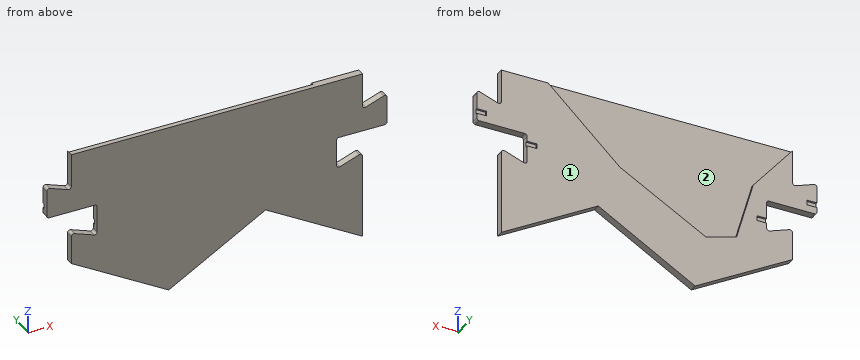
```python
from build123d import *

# Parameters (mm, degrees)
P_IDAT_VYSUNUT_M1_DEPTH  = 3
P_IDAT_VYSUNUT_M2_DEPTH  = 2
ZAOBLIT3_R               = 1
SKICA2_W                 = 4
SKICA2_H                 = 2
ODEBRAT_VYSUNUT_M1_DEPTH = 0.8
SKICA3_W                 = 4
SKICA3_H                 = 2
ODEBRAT_VYSUNUT_M2_DEPTH = 0.8


with BuildPart() as part:
    # Skica1 → P_idat vysunut_m1 (new body)
    with BuildSketch(Plane(origin=(0, 0, 0), x_dir=(1, 0, 0), z_dir=(0, 1, 0))):
        Polygon((-118.143750166, 15), (-118.143750166, 0), (-102.227105248, 19.278496169), (-95.473037065, 43.348863075), (-82.997228437, 47.003202833), (-48.112980408, 27.430537213), (-19, 0), (0, 0), (0, 15), (9.950504516, 11.37831254), (9.950504516, 24.27831254), (-10.5, 24.27831254), (-10.5, 37.37831254), (0, 33.55662508), (0, 69.224902673), (-39.317553332, 46.524902673), (-78.635106664, 69.224902673), (-118.143185584, 46.414902673), (-118.143185584, 33.5570142), (-107.643750166, 37.378496169), (-107.643750166, 24.278496169), (-128.093750166, 24.278496169), (-128.093750166, 11.378496169), align=None)
    extrude(amount=P_IDAT_VYSUNUT_M1_DEPTH)

    # Skica1_3 → P_idat vysunut_m2 (add)
    with BuildSketch(Plane(origin=(0, 0, 0), x_dir=(1, 0, 0), z_dir=(0, 1, 0))):
        Polygon((-102.227105248, 19.278496169), (-118.143750166, 0), (-19, 0), (-48.112980408, 27.430537213), (-82.997228437, 47.003202833), (-95.473037065, 43.348863075), align=None)
    extrude(amount=P_IDAT_VYSUNUT_M2_DEPTH)

    # Zaoblit3
    zaoblit3_edges = [part.edges().sort_by_distance(p)[0] for p in [
        (-10.5, 1.5, -24.27831254),
        (9.950504516, 1.5, -24.27831254),
        (9.950504516, 1.5, -11.37831254),
        (0, 1.5, -15),
        (-118.143750166, 1.5, -15),
        (-128.093750166, 1.5, -11.378496169),
        (-128.093750166, 1.5, -24.278496169),
        (-107.643750166, 1.5, -24.278496169),
        (-107.643750166, 1.5, -37.378496169),
        (-118.143185584, 1.5, -33.5570142),
        (0, 1.5, -33.55662508),
        (-10.5, 1.5, -37.37831254),
    ]]
    fillet(zaoblit3_edges, radius=ZAOBLIT3_R)

    # Skica2 → Odebrat vysunut_m1 (cut)
    with BuildSketch(Plane(origin=(0, 3, 0), x_dir=(1, 0, 0), z_dir=(0, 1, 0))):
        with Locations((-105.643750166, 32.914422166)):
            Rectangle(SKICA2_W, SKICA2_H)
        with Locations((-126.093750166, 20.342570172)):
            Rectangle(SKICA2_W, SKICA2_H)
    extrude(amount=-ODEBRAT_VYSUNUT_M1_DEPTH, mode=Mode.SUBTRACT)

    # Skica3 → Odebrat vysunut_m2 (cut)
    with BuildSketch(Plane(origin=(0, 3, 0), x_dir=(1, 0, 0), z_dir=(0, 1, 0))):
        with Locations((-12.5, 28.314238537)):
            Rectangle(SKICA3_W, SKICA3_H)
        with Locations((7.950504516, 20.342386544)):
            Rectangle(SKICA3_W, SKICA3_H)
    extrude(amount=-ODEBRAT_VYSUNUT_M2_DEPTH, mode=Mode.SUBTRACT)


solid = part.part
```
Input: part model. Units: mm. Frame: model coordinates. Face numbers are marked on the shaded views. Round coordinates to 2 decimals unless told otherwise and drop trailing zeros. Loops run counter-clockwise (first coordinate to the right, second up) from the corner with the lowest first, then second, coordinate; pieces in that order, holes last. Notation, with made-up numbers: M 56.5,44.25 L 114.5,44.25 A16 ccw 114.5,63.25 Z; hole C 67,62.5 d5. An arc over 180 degrees is marked long. Answer in a Markdown table with one row per item. Add a question column.
1. Mould query, pull axis X, two halves, no side actions, for the marked faces 1 and 2. Classes: released by +X, released by -X, zero draft, split by the parting line, or undercut.
2. Contact query for flat-ended pins moving along their axis: pin 1 (1.5 mm diameter, centred on x = -3.5, y = 1.5, fed in from -Z); pin 2 (1.5 mm diameter, centred on y = 2, z = -32, fed in from +X); pin 3 (1 mm diameter, centred on y = 1, z = -24.5, fed in from +X). Output: stop coordinate, or through.
3. Section D-D (z = -17). Output: boundary loops of the cut face in (x, y), and give its area (3 significant figures).
4. Section B-B (z = -48.5). Output: boundary loops of the cut face in (x, y), and give its area (3 significant figures).
5. Section C-C (x = -3). Output: boundary loops of the cut face in (y, z).
6. Ray query, probe 1 along X at (y, z) = (1.25, -27.5); probe 2 along X at (y, z) = (1.05, -11.5); probe 3 along Y at (x, z) = (-54, -18). Return the intervals inside material, ascending.
Values follow:
| question | item | result |
|---|---|---|
| 1 | face 1 | zero draft |
| 1 | face 2 | undercut |
| 2 | pin 1 | z = -67.64 |
| 2 | pin 2 | x = -10.5 |
| 2 | pin 3 | x = 9.64 |
| 3 | outline | M -128.09,0 L 9.95,0 L 9.95,3 L -37.04,3 L -37.04,2 L -104.11,2 L -104.11,3 L -128.09,3 Z |
| 3 | area | 347 mm^2 |
| 4 | outline | M -114.53,0 L -42.74,0 L -42.74,3 L -114.53,3 Z; M -35.9,0 L 0,0 L 0,3 L -35.9,3 Z |
| 4 | area | 323 mm^2 |
| 5 | outline | M 0,-67.49 L 3,-67.49 L 3,-34.65 L 0,-34.65 Z; M 0,-24.28 L 3,-24.28 L 3,0 L 0,0 Z |
| 6 | probe 1 | -107.64 to -10.5 |
| 6 | probe 2 | -118.14 to 0 |
| 6 | probe 3 | 0 to 2 |
